```python
from build123d import *

# Parameters (mm, degrees)
SKETCH_W        = 19.05
SKETCH_H        = 9.525
PAD_DEPTH       = 533.4
SKETCH001_W     = 9.525
SKETCH001_H     = 2.38125
POCKET_DEPTH    = 533.401
SKETCH002_W     = 14.2875
SKETCH002_H     = 3.175
POCKET001_DEPTH = 533.401
SKETCH003_W     = 11.1125
SKETCH003_H     = 1.5875
POCKET002_DEPTH = 533.401


with BuildPart() as part:
    # Sketch → Pad (new body)
    with BuildSketch(Plane.XZ):
        Rectangle(SKETCH_W, SKETCH_H)
    extrude(amount=PAD_DEPTH)

    # Sketch001 (on Face6 of Pad) → Pocket (cut, through all)
    with BuildSketch(Plane.XZ.offset(533.4)):
        with Locations((0, 3.571875)):
            Rectangle(SKETCH001_W, SKETCH001_H)
    extrude(amount=-POCKET_DEPTH, mode=Mode.SUBTRACT)

    # Sketch002 (on Face5 of Pocket) → Pocket001 (cut, through all)
    with BuildSketch(Plane.XZ.offset(533.4)):
        with Locations((0, 0.79375)):
            Rectangle(SKETCH002_W, SKETCH002_H)
    extrude(amount=-POCKET001_DEPTH, mode=Mode.SUBTRACT)

    # Sketch003 (on Face5 of Pocket001) → Pocket002 (cut, through all)
    with BuildSketch(Plane.XZ.offset(533.4)):
        with Locations((0, -1.5875)):
            Rectangle(SKETCH003_W, SKETCH003_H)
    extrude(amount=-POCKET002_DEPTH, mode=Mode.SUBTRACT)


solid = part.part
```
For this review, take the finished solid that the model builds, in its own axes (mm). Round coordinates to 2 decimals unless told otherwise and drop trailing zeros. Loops run counter-clockwise (first coordinate to the right, second up) from the corner with the lowest first, then second, coordinate; pieces in that order, holes last.
(1) Wall thickness on line 1 along X through (y, z) = (-133, -0.75) (3 decimals); line 2 along X through (y, z) = (-191.5, -1.5) (3 decimals); line 3 along Z through (x, y) = (-5.25, -100.5): over which ranges is each line inside the solid? List them lowest first.
Returned:
line 1: x = -9.525 to -7.144, 7.144 to 9.525
line 2: x = -9.525 to -5.556, 5.556 to 9.525
line 3: z = -4.76 to -2.38, 2.38 to 4.76
(2) Clearance check with flat-ended pins moving along their axes: P1, Ø9, axis at x = -0.5, y = -211, coming from the +Z side; P2, Ø8, axis at x = -0.5, y = -182, coming from the +Z side; P3, Ø5, axis at x = -2, z = 1.5, coming from the -Y side. State where each tip first meets the part, or that it passes through.
Returned:
P1: stops at z = 4.76
P2: stops at z = -2.38
P3: passes through
(3) Mouldability with a two-part tool opening along X and no side actions: class faces 1 (the flat face through (9.525, -263, 0)), 2 (the flat face through (0, -533.4, -3)), 3 (the flat face through (0, -270, -2.381)) as released by +X, released by -X, zero draft, split by the parting line, or undercut.
Returned:
face 1: released by +X
face 2: zero draft
face 3: undercut
(4) We need section B-B (x = -1). Give the boundary of the cut face in (y, z).
Returned:
outline: (-533.4, -4.76) - (0, -4.76) - (0, -2.38) - (-533.4, -2.38) - close
(5) We need section A-A (y = -381). Give the boundary of the cut face in (x, z) (1 decimal), plus the area to 3 significant figures.
Returned:
outline: (-9.5, -4.8) - (9.5, -4.8) - (9.5, 4.8) - (4.8, 4.8) - (4.8, 2.4) - (7.1, 2.4) - (7.1, -0.8) - (5.6, -0.8) - (5.6, -2.4) - (-5.6, -2.4) - (-5.6, -0.8) - (-7.1, -0.8) - (-7.1, 2.4) - (-4.8, 2.4) - (-4.8, 4.8) - (-9.5, 4.8) - close
area: 95.8 mm2
